Study the drawing (mm; zero at the part's minimum x, y, z) and answer. A direction names the side the tool comes from. Coordinates: 2 decimals unless noted, no trailing zeros. Order: outer loops, then holes, each group sorted by start corner. A loop starts at its lowest first (then second) coordinate and runs counter-clockwise, first axis right, second up. Notation, with made-up numbers: (-32, 64.5) -> (1, 64.5) arc R26 cw to (1, 101.5) -> close; hole circle Ø6 at (85.25, -6.5). An arc over 180 degrees is marked (long way). Answer as CSV lines item,"result". Start each with the question number.
Item 1: Section B-B (x = 13.5) is taken. Write down the section's boundary in (y, z) (1 decimal).
Item 2: Straight lines are drawn through the part: L1, parallel to X at y = 3.5, z = 9.5; L2, parallel to Y at x = 5.25, z = 10; L3, parallel to Y at x = 1.5, z = 1.5 (1 decimal). For each, find the intervals that lie inside material, in ascending order.
Item 3: Which of the six approach directions +Z, -Z, +X, -X, +Y, -Y give full straight-line access (tool end or side, diameter ignored) to the marked faces 1 and 2?
Item 4: Each of these flat-tipped pins is pushed along its axis until it touches: pin 1 Ø1.5 at (y, z) = (3.5, 9.5) entering from +X; pin 2 Ø4 at (x, y) = (9.5, 13) entering from -Z (1 decimal); pin 3 Ø6 at (x, z) = (12, 8) entering from +Y. Where does it stop, or does it pass through?
Item 5: Section A-A (x = 4) is taken. Write down the section's boundary in (y, z).
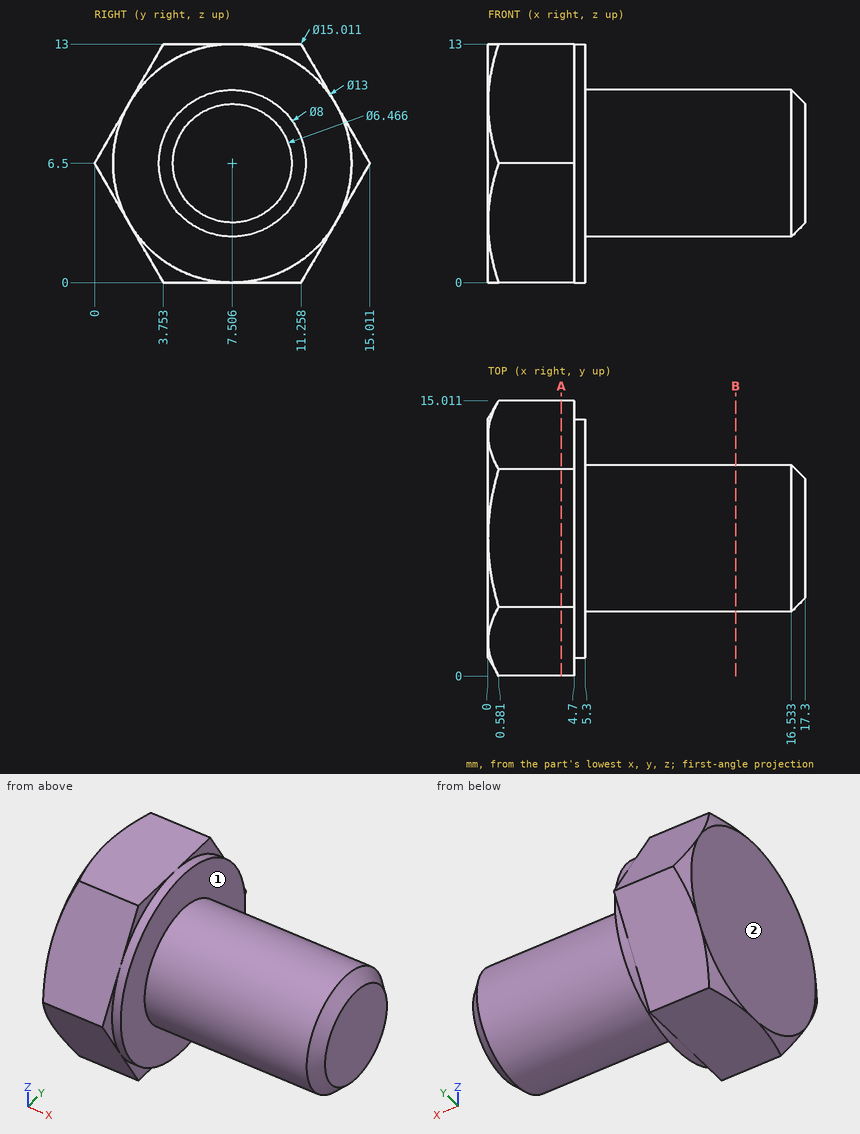
Checked values:
1,outline,"circle Ø8 at (7.5, 6.5)"
2,L1,"x = 0 to 5.3"
2,L2,"y = 2.03 to 12.98"
2,L3,"y = 2.9 to 12.1"
3,face 1,"+X"
3,face 2,"+Z, -Z, -X, +Y, -Y"
4,pin 1,"stops at x = 5.3"
4,pin 2,"stops at z = 4.6"
4,pin 3,"stops at y = 11.51"
5,outline,"(0, 6.5) -> (3.75, 0) -> (11.26, 0) -> (15.01, 6.5) -> (11.26, 13) -> (3.75, 13) -> close"
